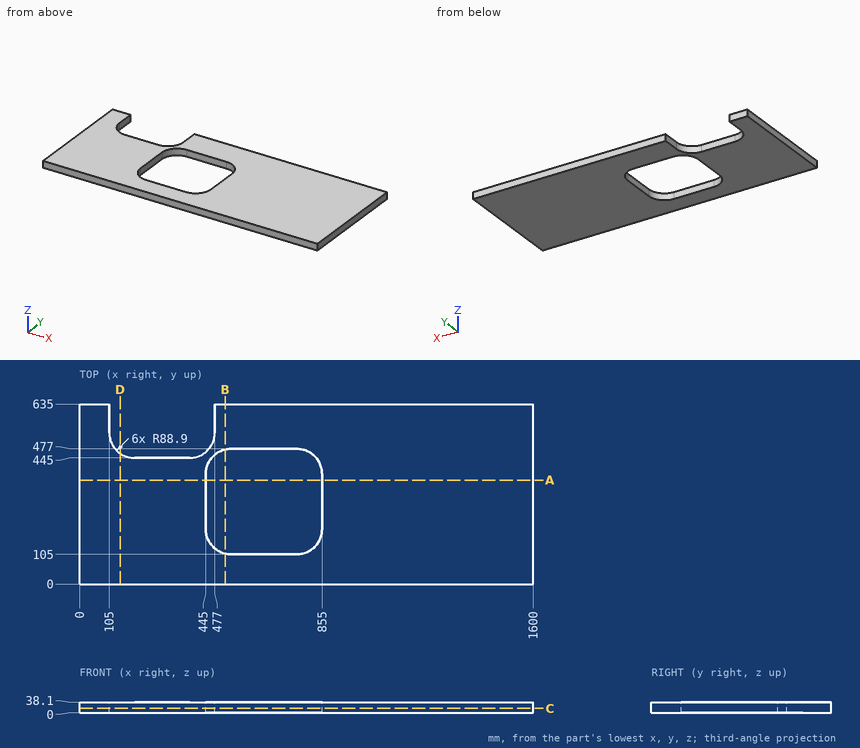
Job drawing, mm, ordinate dimensions from the low corner. One solid piece. Give positions to 0.01 mm unless a question says otherwise; leave off trailing zeros. Loops run counter-clockwise (first coordinate to the right, second up) from the corner with the lowest first, then second, coordinate; pieces in that order, holes last. Notation, with made-up numbers: M 49,-34.5 L 83,-34.5 A22 ccw 83,-9.5 Z; hole C 15.5,75 d2. An arc over 180 degrees is marked long. Use one line per item in the form item = value.
Item 1: Slice it at A-A on y = 367. List the corners of the cut face in (x, z).
Filled in:
outline = M 0,0 L 445,0 L 445,38.1 L 0,38.1 Z; M 855,0 L 1600,0 L 1600,38.1 L 855,38.1 Z
Item 2: Slice it at B-B on x = 513. List the corners of the cut face in (y, z), and give its area (3 significant figures).
Filled in:
outline = M 0,0 L 107.49,0 L 107.49,38.1 L 0,38.1 Z; M 474.51,0 L 635,0 L 635,38.1 L 474.51,38.1 Z
area = 10,200 mm^2
Item 3: Slice it at D-D on x = 143.5. List the corners of the cut face in (y, z).
Filled in:
outline = M 0,0 L 460.67,0 L 460.67,38.1 L 0,38.1 Z
Item 4: Slice it at C-C on z = 16.5. List the corners of the cut face in (x, y).
Filled in:
outline = M 0,0 L 1600,0 L 1600,635 L 477,635 L 477,533.9 A88.9 cw 388.1,445 L 193.9,445 A88.9 cw 105,533.9 L 105,635 L 0,635 Z; hole M 445,193.9 A88.9 ccw 533.9,105 L 766.1,105 A88.9 ccw 855,193.9 L 855,388.1 A88.9 ccw 766.1,477 L 533.9,477 A88.9 ccw 445,388.1 Z
Item 5: Flat gauge pin, fed straight in: pin 1 Ø2 at (x, z) = (334, 7) entering from +Y. Where does the tip first touch, or does it go through?
Filled in:
pin_1 = 445
Item 6: Drill centre lines: L1, parallel to X at y = 361, z = 12; L2, parallel to X at y = 543.5, z = 6.5; L3, parallel to Y at x = 542, z = 2.5. Where is each one in solid material? Low to high.
Filled in:
L1 = 0 to 445, 855 to 1600
L2 = 0 to 105, 477 to 1600
L3 = 0 to 105, 477 to 635
